```python
from build123d import *

# Parameters (mm, degrees)
SKETCH_1_R             = 6
EXTRUDE_1_DEPTH        = 76
HOLE_WIZARD_M6_1_D     = 5
HOLE_WIZARD_M6_1_DEPTH = 33
HOLE_WIZARD_M6_1_TIP   = 1.502151548
HOLE_WIZARD_M6_2_D     = 5
HOLE_WIZARD_M6_2_DEPTH = 33
HOLE_WIZARD_M6_2_TIP   = 1.502151548


with BuildPart() as part:
    # 草图1 → 凸台-拉伸1 (new body)
    with BuildSketch(Plane.XY):
        Circle(SKETCH_1_R)
    extrude(amount=EXTRUDE_1_DEPTH)

    # M6 螺纹孔1
    with Locations(Plane.XY.offset(76)):
        with Locations((0, 0)):
            Hole(HOLE_WIZARD_M6_1_D / 2, depth=HOLE_WIZARD_M6_1_DEPTH)
            with Locations((0, 0, -(HOLE_WIZARD_M6_1_DEPTH + HOLE_WIZARD_M6_1_TIP / 2))):  # 118° drill point
                Cone(0, HOLE_WIZARD_M6_1_D / 2, HOLE_WIZARD_M6_1_TIP, mode=Mode.SUBTRACT)

    # M6 螺纹孔2
    with Locations(Plane(origin=(0, 0, 0), x_dir=(-1, 0, 0), z_dir=(0, 0, -1))):
        with Locations((0, 0)):
            Hole(HOLE_WIZARD_M6_2_D / 2, depth=HOLE_WIZARD_M6_2_DEPTH)
            with Locations((0, 0, -(HOLE_WIZARD_M6_2_DEPTH + HOLE_WIZARD_M6_2_TIP / 2))):  # 118° drill point
                Cone(0, HOLE_WIZARD_M6_2_D / 2, HOLE_WIZARD_M6_2_TIP, mode=Mode.SUBTRACT)


solid = part.part
```
The model under review builds one solid part; all positions refer to its coordinate system, in mm. A direction names the side the tool comes from. Coordinates: 2 decimals unless noted, no trailing zeros. Order: outer loops, then holes, each group sorted by start corner. A loop starts at its lowest first (then second) coordinate and runs counter-clockwise, first axis right, second up. Notation, with made-up numbers: M 68.25,63.5 L 113.25,63.5 A27 ccw 113.25,82.5 Z; hole C -21,-30 d6. An arc over 180 degrees is marked long. One line per question, with ' | ' between items.
(1) The part is to be moulded in two halves that separate along X. For faces 4 (the face through (3, 0, 0)), 5 (the face through (-6, 0, 37)), 6 (the face through (0.094, -0.424, 34.241)), say which applies: +X half, -X half, draft (parallel to the pull), parting line (faces both ways), or undercut.
Geometry results:
face 4: draft | face 5: parting line | face 6: undercut
(2) Machinability: for faces 1 (the face through (3, 0, 76)), 2 (the face through (0.54, -2.44, 59.27)), 3 (the face through (-0.54, -2.44, 16.73)), which of the approach directions +Z, -Z, +X, -X, +Y, -Y give a long, thin tool a straight path to every point of the face, cutting with its end or side? Answer none if there is none.
Geometry results:
face 1: +Z, +X, -X, +Y, -Y | face 2: +Z | face 3: -Z
(3) Add section B-B, the plane z = 38. Write out the cut boundary in (x, y).
Geometry results:
outline: C 0,0 d12
(4) Add section C-C, the plane y = -3.25. Write out the cut boundary in (x, z), then the cut area to 3 significant figures.
Geometry results:
outline: M -5.04,0 L 5.04,0 L 5.04,76 L -5.04,76 Z | area: 767 mm²
(5) Add section D-D, the plane x = 5. Write out the cut boundary in (y, z), then the cut area to 3 significant figures.
Geometry results:
outline: M -3.32,0 L 3.32,0 L 3.32,76 L -3.32,76 Z | area: 504 mm²
(6) Add section A-A, the plane z = 6.5. Write out the cut boundary in (x, y), then the cut area to 3 significant figures.
Geometry results:
outline: C 0,0 d12; hole C 0,0 d5 | area: 93.5 mm²
(7) For probe 1 along Y at (x, z) = (0.25, 11); probe 2 along X at (y, z) = (1.5, 20.5); probe 3 along Y at (x, z) = (2, 57.5), list the stretches that pass through material, from the lowest coordinate up. Write a range as from..to.
Geometry results:
probe 1: y = -5.99..-2.49, 2.49..5.99 | probe 2: x = -5.81..-2, 2..5.81 | probe 3: y = -5.66..-1.5, 1.5..5.66
(8) Insertion check: pin 1 (3 mm diameter, centred on y = 3.5, z = 38.5, fed in from -X); pin 2 (4.5 mm diameter, centred on x = 0, y = 0, fed in from +Z); pin 3 (1.5 mm diameter, centred on y = -3.5, z = 27.5, fed in from -X). Each pin has a flat end and moves straight along its axis. Give the tip position at first contact, or say it passes through.
Geometry results:
pin 1: stops at x = -5.66 | pin 2: stops at z = 42.85 | pin 3: stops at x = -5.33
